```python
from build123d import *

# Parameters (mm, degrees)
ESQUISSE1_W                      = 48
ESQUISSE1_H                      = 45
BOSS_EXTRU_1_DEPTH               = 8
ESQUISSE5_R                      = 5.5
ENL_V_MAT_EXTRU_3_DEPTH          = 2
ESQUISSE4_R                      = 8.25
ENL_V_MAT_EXTRU_4_DEPTH          = 6
ESQUISSE2_R                      = 1.75
ENL_V_MAT_EXTRU_5_DEPTH          = 10
D_GAGEMENT_M3_51_D               = 3.7
D_GAGEMENT_M3_51_DEPTH           = 10
D_GAGEMENT_M3_51_TIP             = 1.111592145
D_GAGEMENT_M3_51_ON_FACE_2_D     = 3.7
D_GAGEMENT_M3_51_ON_FACE_2_DEPTH = 10
D_GAGEMENT_M3_51_ON_FACE_2_TIP   = 1.111592145


with BuildPart() as part:
    # Esquisse1 → Boss.-Extru.1 (new body)
    with BuildSketch(Plane.XY):
        Rectangle(ESQUISSE1_W, ESQUISSE1_H)
    extrude(amount=BOSS_EXTRU_1_DEPTH)

    # Esquisse5 → Enlèv. mat.-Extru.3 (cut)
    with BuildSketch(Plane.XY.offset(8)):
        with Locations((0, -4.5)):
            Circle(ESQUISSE5_R)
    extrude(amount=-ENL_V_MAT_EXTRU_3_DEPTH, mode=Mode.SUBTRACT)

    # Esquisse4 → Enlèv. mat.-Extru.4 (cut)
    with BuildSketch(Plane(origin=(0, 0, 0), x_dir=(-1, 0, 0), z_dir=(0, 0, -1))):
        with Locations((0, -4.5)):
            Circle(ESQUISSE4_R)
    extrude(amount=-ENL_V_MAT_EXTRU_4_DEPTH, mode=Mode.SUBTRACT)

    # Esquisse2 → Enlèv. mat.-Extru.5 (cut)
    with BuildSketch(Plane.XZ.offset(22.5)):
        with Locations((-20, 4)):
            Circle(ESQUISSE2_R)
        with Locations((20, 4)):
            Circle(ESQUISSE2_R)
    extrude(amount=-ENL_V_MAT_EXTRU_5_DEPTH, mode=Mode.SUBTRACT)

    # Dégagement M3.51
    with Locations(Plane(origin=(20, 22.5, 4), x_dir=(0, 0, 1), z_dir=(0, 1, 0))):
        with Locations((0, 0), (0, -40)):
            Hole(D_GAGEMENT_M3_51_D / 2, depth=D_GAGEMENT_M3_51_DEPTH)
            with Locations((0, 0, -(D_GAGEMENT_M3_51_DEPTH + D_GAGEMENT_M3_51_TIP / 2))):  # 118° drill point
                Cone(0, D_GAGEMENT_M3_51_D / 2, D_GAGEMENT_M3_51_TIP, mode=Mode.SUBTRACT)

    # Dégagement M3.51 on face 2
    with Locations(Plane(origin=(-58.361225935, 70.859654688, 0), x_dir=(0, 0, 1), z_dir=(0, 1, 0))):
        with Locations((0, 0)):
            Hole(D_GAGEMENT_M3_51_ON_FACE_2_D / 2, depth=D_GAGEMENT_M3_51_ON_FACE_2_DEPTH)
            with Locations((0, 0, -(D_GAGEMENT_M3_51_ON_FACE_2_DEPTH + D_GAGEMENT_M3_51_ON_FACE_2_TIP / 2))):  # 118° drill point
                Cone(0, D_GAGEMENT_M3_51_ON_FACE_2_D / 2, D_GAGEMENT_M3_51_ON_FACE_2_TIP, mode=Mode.SUBTRACT)


solid = part.part
```
Build history of the part. All positions in model axes, mm. A direction names the side the tool comes from. Give positions to 0.01 mm unless a question says otherwise; leave off trailing zeros. Loops run counter-clockwise (first coordinate to the right, second up) from the corner with the lowest first, then second, coordinate; pieces in that order, holes last. Notation, with made-up numbers: (40, 28.25) -> (68, 28.25) arc R10 cw to (68, 33.25) -> close; hole circle Ø10 at (68.25, -16). An arc over 180 degrees is marked (long way). One line per question, with ' | ' between items.
Q1. Cut at A-A, the plane y = -4.5. Write the cut outline in (x, z).
Filled sheet:
outline: (-24, 0) -> (-8.25, 0) -> (-8.25, 6) -> (-5.5, 6) -> (-5.5, 8) -> (-24, 8) -> close; (5.5, 6) -> (8.25, 6) -> (8.25, 0) -> (24, 0) -> (24, 8) -> (5.5, 8) -> close
Q2. Tool access for faces 4 (the flat face through (-2, -10, 6)), 5 (the flat face through (0, 22.5, 4)), 6 (the cylindrical face through (-18.166, 17.43, 4.241)), 7 (the flat face through (-20, -12.5, 4)): list every direction of +Z, -Z, +X, -X, +Y, -Y with a clear straight run to the whole face (end or side of a thin tool).
Filled sheet:
face 4: -Z | face 5: +Z, -Z, +X, -X, +Y | face 6: +Y | face 7: -Y
Q3. Cut at C-C, the plane y = -19.5. Write the cut outline in (x, z), plus the area to 3 significant figures.
Filled sheet:
outline: (-24, 0) -> (24, 0) -> (24, 8) -> (-24, 8) -> close; hole circle Ø3.5 at (-20, 4); hole circle Ø3.5 at (20, 4) | area: 365 mm²
Q4. Drill centre lines: line 1 along X through (y, z) = (15, 4); line 2 along Z through (x, y) = (-20, 18.5); line 3 along Y through (x, z) = (0, 6.9). Where is each one in solid material? Low to high. Write a range as [from, to].
Filled sheet:
line 1: x = [-24, -21.85], [-18.15, 18.15], [21.85, 24] | line 2: z = [0, 2.15], [5.85, 8] | line 3: y = [-22.5, -10], [1, 22.5]
Q5. Cut at B-B, the plane x = 0. Write the cut outline in (y, z), plus the area to 3 significant figures.
Filled sheet:
outline: (-22.5, 0) -> (-12.75, 0) -> (-12.75, 6) -> (-10, 6) -> (-10, 8) -> (-22.5, 8) -> close; (1, 6) -> (3.75, 6) -> (3.75, 0) -> (22.5, 0) -> (22.5, 8) -> (1, 8) -> close | area: 239 mm²
Q6. Pull direction Z, two halves, no side cores. Call faces 1 (the cylindrical face through (-21.75, -17.57, 4.08)), 2 (the flat face through (0, 5, 0)), 3 (the flat face through (-24, 0, 4)): pulls with the +Z half, pulls with the -Z half, needs draft (parallel to the pull), parting line crosses it, or undercut.
Filled sheet:
face 1: undercut | face 2: pulls with the -Z half | face 3: needs draft
Q7. Drop flat-ended pins along their axis: pin 1 (3 mm diameter, centred on x = 20, z = 4, fed in from -Y); pin 2 (5 mm diameter, centred on x = 2, y = -8, fed in from -Z). Give the stop position or say it passes through.
Filled sheet:
pin 1: stops at y = -12.5 | pin 2: stops at z = 6
Q8. Cut at D-D, the plane y = 3. Write the cut outline in (x, z).
Filled sheet:
outline: (-24, 0) -> (-3.44, 0) -> (-3.44, 6) -> (3.44, 6) -> (3.44, 0) -> (24, 0) -> (24, 8) -> (-24, 8) -> close
